Source: CAD feature listing. Evaluate the final solid. Frame: model axes, mm. A direction names the side the tool comes from. Round coordinates to 2 decimals unless told otherwise and drop trailing zeros. Loops run counter-clockwise (first coordinate to the right, second up) from the corner with the lowest first, then second, coordinate; pieces in that order, holes last.
Item 1: Pull-direction query (Y, two-part tool) for faces 3 (the flat face through (-22.225, 89, 0)), 4 (the flat face through (0, 180.975, 10)), 5 (the cylindrical face through (10.993, 40.777, -11.135)); classes: released by +Y, released by -Y, zero draft, split by the parting line, or undercut.
Item 2: Section query A-A on y = 101.6. Return loops of the section in (x, z) (1 decimal), then the cut area to 3 significant figures.
Item 3: Section query D-D on x = -4. Return loops of the section in (y, z) (3 decimals), then the cut area to 3 significant figures.
Item 4: First-contact query: P1, Ø5, axis at x = -5.5, z = -9, coming from the +Y side (3 decimals). Flat tip, straight axial feed; report the tip coordinate or a pass-through.
Item 5: Section query C-C on z = 2. Return loops of the section in (x, y) (3 decimals), then the cut area to 3 significant figures.
Item 6: Access query for faces 1 (the flat face through (22.225, 89, 0)), 2 (the cylindrical face through (1.86, 169.74, 11.09)). Directions: +Z, -Z, +X, -X, +Y, -Y. A direction counts if a zero-diameter tool reaches every point of the face in a straight line with its end or side. Return the directions, or none.
Item 7: Section query B-B on y = 38.1. Return loops of the section in (x, z) (3 decimals), then the cut area to 3 significant figures.
Item 8: Ray query, L1, parallel to Y at x = 0, z = 11.3 (1 decimal); L2, parallel to Y at x = 1, z = -9.75 (3 decimals); L3, parallel to Z at x = -19, y = 123.5 (3 decimals). Return the intervals inside material, ascending.
Autodesk Inventor part; units mm, degrees
ref_plane "YZ Plane" through (0, 0, 0) normal (1, 0, 0) x (0, 1, 0)
ref_plane "XZ Plane" through (0, 0, 0) normal (0, 1, 0) x (-1, 0, 0)
ref_plane "XY Plane" through (0, 0, 0) normal (0, 0, 1) x (1, 0, 0)
sketch "Sketch1" plane through (0, 0, 0) normal (0, 1, 0) x (-1, 0, 0)
  line L0 (25.4, 12.7) -> (-25.4, 12.7)
  line L1 (-25.4, 12.7) -> (-25.4, -12.7)
  line L2 (-25.4, -12.7) -> (25.4, -12.7)
  line L3 (25.4, -12.7) -> (25.4, 12.7)
  line L4 (25.4, 12.7) -> (-25.4, -12.7) construction
  line L5 (-25.4, 12.7) -> (25.4, -12.7) construction
  line L6 (22.225, 9.525) -> (-22.225, 9.525)
  line L7 (-22.225, 9.525) -> (-22.225, -9.525)
  line L8 (-22.225, -9.525) -> (22.225, -9.525)
  line L9 (22.225, -9.525) -> (22.225, 9.525)
  line L10 (22.225, 9.525) -> (-22.225, -9.525) construction
  line L11 (-22.225, 9.525) -> (22.225, -9.525) construction
  point P0 (0, 0)
  dimension "d0" = 50.8
  dimension "d1" = 25.4
  dimension "d2" = 44.45
  dimension "d3" = 19.05
extrude "Extrusion1" add sketch "Sketch1" along normal blind 180.975
sketch "Sketch2" plane through (25.4, 0, -12.7) normal (0, 0, -1) x (-1, 0, 0)
  line L0 (50.8, 0) -> (50.8, 180.975)
  line L1 (0, 180.975) -> (50.8, 180.975)
  line L2 (0, 0) -> (0, 180.975)
  line L3 (25.4, 0) -> (63.5, 0) construction
  line L4 (25.4, 38.1) -> (50.8, 38.1)
  line L5 (50.8, 38.1) -> (0, 38.1)
  line L6 (0, 38.1) -> (12.7, 38.1)
  line L7 (0, 38.1) -> (12.7, 38.1) construction
  line L8 (12.7, 38.1) -> (38.1, 38.1)
  circle A0 centre (12.7, 38.1) radius 3.175
  circle A1 centre (38.1, 38.1) radius 3.175
  line L9 (25.4, 180.975) -> (25.4, 155.575)
  line L10 (25.4, 180.975) -> (50.8, 180.975) construction
  circle A2 centre (25.4, 155.575) radius 14.2875
  dimension "d6" = 38.1
  dimension "d8" = 12.7
  dimension "d9" = 0
  dimension "d10" = 25.4
  dimension "d11" = 180
  dimension "d12" = 6.35
  dimension "d13" = 6.35
  dimension "d14" = 25.4
  dimension "d15" = 90
  dimension "d16" = 28.575
extrude "Extrusion2" cut sketch "Sketch2" against normal blind 180.975 contours A2 | A1 L4 | L4 A1 | A0 L5 | L5 A0
sketch "Sketch3" plane through (25.4, 0, -12.7) normal (0, 0, -1) x (-1, 0, 0)
  line L0 (0, 0) -> (0, 180.975)
  line L1 (25.4, 0) -> (25.4, 101.6)
  line L2 (25.4, 0) -> (127, 0) construction
  circle A0 centre (25.4, 101.6) radius 14.2875
  line L3 (25.4, 101.6) -> (43.3605, 119.5605)
  line L4 (25.4, 101.6) -> (50.8, 101.6) construction
  line L5 (43.3605, 119.5605) -> (7.4395, 83.6395)
  line L6 (7.4395, 83.6395) -> (43.3605, 83.6395)
  line L7 (43.3605, 83.6395) -> (43.3605, 119.5605)
  line L8 (43.3605, 119.5605) -> (7.4395, 119.5605)
  line L9 (7.4395, 119.5605) -> (7.4395, 83.6395)
  circle A1 centre (7.4395, 119.5605) radius 2.032
  circle A2 centre (43.3605, 119.5605) radius 2.032
  circle A3 centre (43.3605, 83.6395) radius 2.032
  circle A4 centre (7.4395, 83.6395) radius 2.032
  dimension "d19" = 101.6
  dimension "d20" = 90
  dimension "d21" = 28.575
  dimension "d22" = 25.4
  dimension "d23" = 45
  dimension "d24" = 50.8
  dimension "d25" = 0
  dimension "d26" = 4.064
  dimension "d27" = 4.064
  dimension "d28" = 4.064
  dimension "d29" = 4.064
extrude "Extrusion3" cut sketch "Sketch3" against normal blind 180.975 contours A0 L5 L1 | L1 L3 A0 | A4 L9 L6 | L6 L5 A4 | A3 L7 L6 | L6 L7 A3 | L5 A0 L3 | L9 A4 L5 | A1 L8 L9 | L9 L8 A1 | A2 L3 L7 | L7 L8 A2 | A2 L8 L3
properties part number "Z-ArmStructure"
Data:
1. face 3: zero draft
1. face 4: released by +Y
1. face 5: undercut
2. outline: (-25.4, -12.7) - (-14.3, -12.7) - (-14.3, -9.5) - (-22.2, -9.5) - (-22.2, 9.5) - (-14.3, 9.5) - (-14.3, 12.7) - (-25.4, 12.7) - close; (14.3, -12.7) - (25.4, -12.7) - (25.4, 12.7) - (14.3, 12.7) - (14.3, 9.5) - (22.2, 9.5) - (22.2, -9.5) - (14.3, -9.5) - close
2. area: 262 mm2
3. outline: (0, -12.7) - (87.884, -12.7) - (87.884, -9.525) - (0, -9.525) - close; (0, 9.525) - (87.884, 9.525) - (87.884, 12.7) - (0, 12.7) - close; (115.316, -12.7) - (141.859, -12.7) - (141.859, -9.525) - (115.316, -9.525) - close; (115.316, 9.525) - (141.859, 9.525) - (141.859, 12.7) - (115.316, 12.7) - close; (169.291, -12.7) - (180.975, -12.7) - (180.975, -9.525) - (169.291, -9.525) - close; (169.291, 9.525) - (180.975, 9.525) - (180.975, 12.7) - (169.291, 12.7) - close
3. area: 801 mm2
4. P1: stops at y = 180.975
5. outline: (-25.4, 0) - (-22.225, 0) - (-22.225, 180.975) - (-25.4, 180.975) - close; (22.225, 0) - (25.4, 0) - (25.4, 180.975) - (22.225, 180.975) - close
5. area: 1,150 mm2
6. face 1: +Y, -Y
6. face 2: +Z, -Z
7. outline: (-25.4, -12.7) - (-15.875, -12.7) - (-15.875, -9.525) - (-22.225, -9.525) - (-22.225, 9.525) - (-15.875, 9.525) - (-15.875, 12.7) - (-25.4, 12.7) - close; (-9.525, -12.7) - (9.525, -12.7) - (9.525, -9.525) - (-9.525, -9.525) - close; (-9.525, 9.525) - (9.525, 9.525) - (9.525, 12.7) - (-9.525, 12.7) - close; (15.875, -12.7) - (25.4, -12.7) - (25.4, 12.7) - (15.875, 12.7) - (15.875, 9.525) - (22.225, 9.525) - (22.225, -9.525) - (15.875, -9.525) - close
7. area: 363 mm2
8. L1: y = 0 to 87.3, 115.9 to 141.3, 169.9 to 181
8. L2: y = 0 to 87.348, 115.852 to 141.323, 169.827 to 180.975
8. L3: z = -12.7 to -9.525, 9.525 to 12.7
